Input: part model. Units: mm. Frame: model coordinates. A direction names the side the tool comes from. Round coordinates to 2 decimals unless told otherwise and drop trailing zeros. Write each loop counter-clockwise with the first axis right and the second up, starting at its lowest first coordinate (ties: lowest second). Pieces come first, ordered by that corner, then holes. Notation, with made-up numbers: M 7.25,39.5 L 63.25,39.5 A18 cw 63.25,74.5 Z; hole C 86.25,-16 d11. An arc over 180 degrees is marked long. Write each question's results on one line, items separated by ' | '. Start each with the question number.
```python
from build123d import *

# Parameters (mm, degrees)
BASE_FLANGE1_DEPTH = 110
CHAMFER1_SIZE2     = 3
CHAMFER1_SIZE      = 1.5


# Sheet-metal steps are written as plain solids
with BuildPart() as part:
    # Sketch1 → Base-Flange1 (new body)
    with BuildSketch(Plane(origin=(0, 0, 0), x_dir=(1, 0, 0), z_dir=(0, 1, 0))):
        with BuildLine():
            Line((0, 0), (0, -20))
            Line((0, -20), (0, -33.90302477))
            ThreePointArc((0, -33.90302477), (0.006301715, -33.999170363), (0.025099036, -34.093670879))
            Line((0.025099036, -34.093670879), (7.221834227, -60.952252257))
            ThreePointArc((7.221834227, -60.952252257), (7.252805527, -61.043490765), (7.295420878, -61.129906149))
            Line((7.295420878, -61.129906149), (21.198445648, -85.21065143))
            ThreePointArc((21.198445648, -85.21065143), (21.25197589, -85.290765098), (21.315505105, -85.363206285))
            Line((21.315505105, -85.363206285), (40.977351294, -105.025052473))
            ThreePointArc((40.977351294, -105.025052473), (41.04979248, -105.088581688), (41.129906149, -105.14211193))
            Line((41.129906149, -105.14211193), (65.21065143, -119.0451367))
            ThreePointArc((65.21065143, -119.0451367), (65.297066813, -119.087752052), (65.388305321, -119.118723352))
            Line((65.388305321, -119.118723352), (92.246886699, -126.315458542))
            ThreePointArc((92.246886699, -126.315458542), (92.341387215, -126.334255863), (92.437532808, -126.340557578))
            Line((92.437532808, -126.340557578), (106.340557578, -126.340557578))
            Line((106.340557578, -126.340557578), (106.340557578, -127.840557578))
            Line((106.340557578, -127.840557578), (92.437532808, -127.840557578))
            ThreePointArc((92.437532808, -127.840557578), (92.145597926, -127.821423155), (91.858658132, -127.764347281))
            Line((91.858658132, -127.764347281), (65.000076753, -120.567612091))
            ThreePointArc((65.000076753, -120.567612091), (64.723041665, -120.47357135), (64.46065143, -120.344174806))
            Line((64.46065143, -120.344174806), (40.379906149, -106.441150036))
            ThreePointArc((40.379906148, -106.441150036), (40.136650336, -106.278611699), (39.916691122, -106.085712644))
            Line((39.916691122, -106.085712645), (20.254844934, -86.423866456))
            ThreePointArc((20.254844934, -86.423866456), (20.06194588, -86.203907242), (19.899407542, -85.96065143))
            Line((19.899407542, -85.96065143), (5.996382772, -61.879906149))
            ThreePointArc((5.996382772, -61.879906149), (5.866986228, -61.617515913), (5.772945487, -61.340480825))
            Line((5.772945487, -61.340480825), (-1.423789703, -34.481899447))
            ThreePointArc((-1.423789703, -34.481899447), (-1.480865577, -34.194959652), (-1.5, -33.90302477))
            Line((-1.5, -33.90302477), (-1.5, -20))
            Line((-1.5, -20), (-1.5, 0))
            Line((-1.5, 0), (0, 0))
        make_face()
    extrude(amount=BASE_FLANGE1_DEPTH)

    # Chamfer1
    chamfer1_edges = [part.edges().sort_by_distance(p)[0] for p in [
        (106.340557578, 55, 126.340557578),
    ]]
    chamfer1_side = [part.faces().sort_by_distance(p)[0] for p in [
        (106.340557578, 55, 126.370557578),
    ]]
    chamfer(chamfer1_edges, length=CHAMFER1_SIZE - 0.0001, length2=CHAMFER1_SIZE2 - 0.0001, reference=chamfer1_side[0])  # a hair under: the kernel refuses the full size


solid = part.part
```
1. Access query for faces 1 (the face through (98, 54, 126.341)), 2 (the face through (30.22, 54.23, 96.39)). Directions: +Z, -Z, +X, -X, +Y, -Y. A direction counts if a zero-diameter tool reaches every point of the face in a straight line with its end or side. Return the directions, or none.
2. Cut plane B-B on z = 27. Output: boundary loops of the cut face in (x, y), and give its area (3 significant figures).
3. Contact query for flat-ended pins moving along their axis: P1, Ø5.5, axis at x = 96, y = 34.5, coming from the -Z side; P2, Ø1.5, axis at x = 42, y = 61.5, coming from the +Z side; P3, Ø4, axis at x = 18, y = 52, coming from the -Z side. Output: stop coordinate, or through.
4. Cut plane C-C on x = 95.5. Output: boundary loops of the cut face in (y, z), and give its area (3 significant figures).
5. Line query: L1, parallel to X at y = 49, z = 9.5; L2, parallel to Z at x = 98, y = 47; L3, parallel to Z at x = 30, y = 79. Output: solid intervals per line, ascending. Write a range as from..to.
Answers follow:
1) face 1: -Z, +X, +Y, -Y | face 2: +Z, -X, +Y, -Y
2) outline: M -1.5,0 L 0,0 L 0,110 L -1.5,110 Z | area: 165 mm2
3) P1: stops at z = 126.34 | P2: stops at z = 107.81 | P3: stops at z = 76.21
4) outline: M 0,126.34 L 110,126.34 L 110,127.84 L 0,127.84 Z | area: 165 mm2
5) L1: x = -1.5..0 | L2: z = 126.34..127.84 | L3: z = 94.05..96.17
